Geometry: see drawing. Coordinates: mm, zero at the bounding-box minimum. A direction names the side the tool comes from. Give positions to 0.01 mm unless a question says otherwise; leave off trailing zeros. Order: outer loops, then holes, each group sorted by start corner. A loop starts at its lowest first (then second) coordinate and runs counter-clockwise, first axis right, second up. Notation, with made-up numbers: M 27.25,87 L 68.25,87 A27 cw 68.25,116 Z; hole C 4.25,55.5 d1. An arc over 180 degrees is marked long. Answer as a JSON object with one key per item and string values. Group by question number.
1. Set-up query: the marked faces 1 and 2. Return all of +Z, -Z, +X, -X, +Y, -Y with unobstructed straight access to the full face (end or side cutting, diameter ignored); none if empty.
2. Material intervals for L1, parallel to Z at x = 19, y = 5.5; L2, parallel to X at y = 12.5, z = 46.5; L3, parallel to X at y = 5, z = 48, sorted ascending. Write a range as [from, to].
3. Section query B-B (x = 21). Output: boundary loops of the cut face in (y, z), plus the area to 3 significant figures.
4. Section query A-A (y = 7.5). Output: boundary loops of the cut face in (x, z).
5. Section query D-D (x = 5.25). Output: boundary loops of the cut face in (y, z).
6. Pin query (flat end, axial travel): P1, Ø4, axis at y = 10, z = 9.5, coming from the -X side; P2, Ø5, axis at x = 15, y = 6.5, coming from the -Z side; P3, Ø4, axis at x = 19.5, y = 8, coming from the -Z side; P4, Ø6, axis at x = 14.5, y = 3.5, coming from the +Z side. Return the tip coordinate at first contact, or that it passes through.
7. Section query C-C (z = 17). Output: boundary loops of the cut face in (x, y).
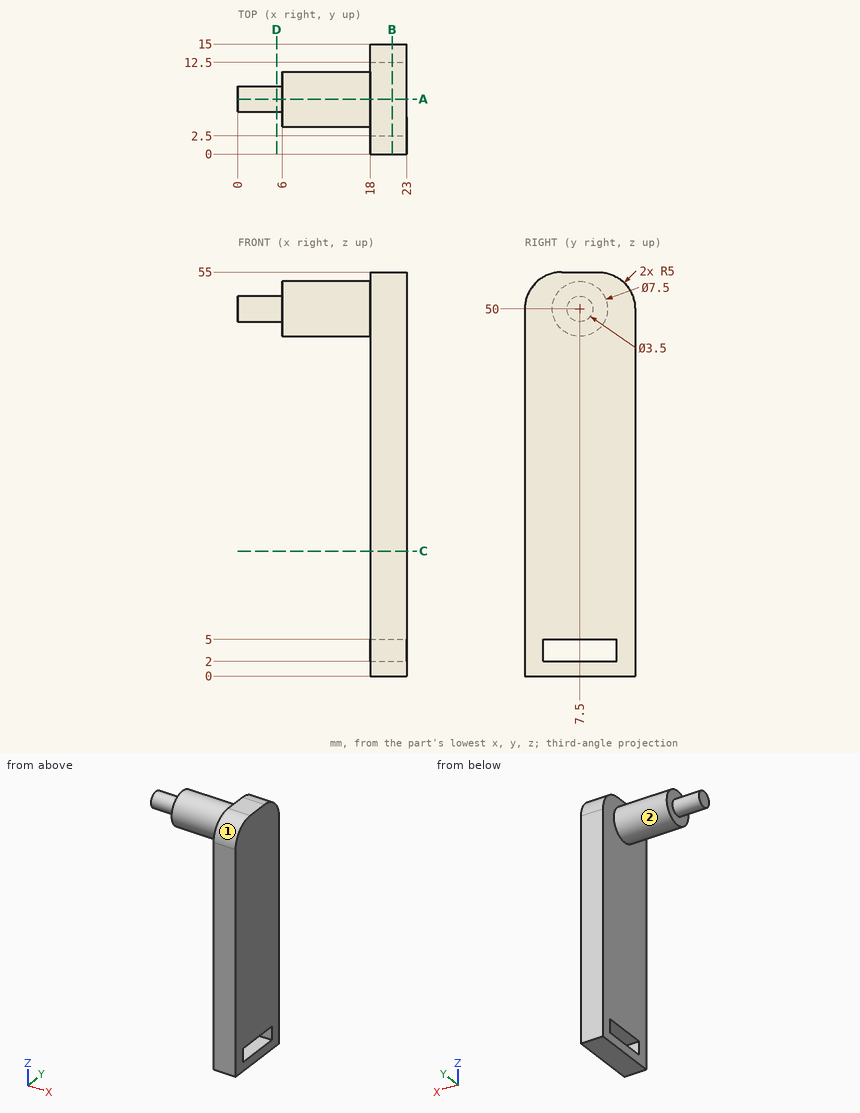
Answer sheet:
{
 "1": {"face 1": "+Z, +X, -X, -Y", "face 2": "-X"},
 "2": {"L1": "[0, 2], [5, 55]", "L2": "[18, 23]", "L3": "[6, 23]"},
 "3": {"outline": "M 0,0 L 15,0 L 15,50 A5 ccw 10,55 L 5,55 A5 ccw 0,50 Z; hole M 2.5,2 L 12.5,2 L 12.5,5 L 2.5,5 Z", "area": "784 mm^2"},
 "4": {"outline": "M 0,48.25 L 6,48.25 L 6,46.25 L 18,46.25 L 18,5 L 23,5 L 23,55 L 18,55 L 18,53.75 L 6,53.75 L 6,51.75 L 0,51.75 Z; M 18,0 L 23,0 L 23,2 L 18,2 Z"},
 "5": {"outline": "C 7.5,50 d3.5"},
 "6": {"P1": "x = 18", "P2": "z = 46.25", "P3": "z = 0", "P4": "z = 53.61"},
 "7": {"outline": "M 18,0 L 23,0 L 23,15 L 18,15 Z"}
}
